from build123d import *

# Parameters (mm, degrees)
SKETCH2_R          = 3.5
CUT_EXTRUDE1_DEPTH = 69.058798109
SKETCH3_R          = 7
CUT_EXTRUDE2_DEPTH = 10
SKETCH3_3_R        = 2.5
CUT_EXTRUDE3_DEPTH = 72.637978754
FILLET1_R          = 1


with BuildPart() as part:
    # Sketch1 → Revolve1 (revolve)
    with BuildSketch(Plane(origin=(0, 0, 0), x_dir=(0, 0, -1), z_dir=(1, 0, 0))):
        Polygon((0, 33), (-14, 33), (-14, 46), (6, 46), (6, 12), (16, 12), (16, 0), (0, 0), align=None)
    revolve(axis=Axis((0, 0, -16), (0, 0, 1)))

    # Sketch2 → Cut-Extrude1 (cut, through all)
    with BuildSketch(Plane(origin=(0, 0, -6), x_dir=(-1, 0, 0), z_dir=(0, 0, -1))):
        with Locations(Location((19.5, -33.774990748, 0), (0, 0, 90))):
            Circle(SKETCH2_R)
        with Locations(Location((-19.5, -33.774990748, 0), (0, 0, 90))):
            Circle(SKETCH2_R)
        with Locations(Location((-39, 0, 0), (0, 0, 90))):
            Circle(SKETCH2_R)
        with Locations(Location((-19.5, 33.774990748, 0), (0, 0, 90))):
            Circle(SKETCH2_R)
        with Locations(Location((19.5, 33.774990748, 0), (0, 0, 90))):
            Circle(SKETCH2_R)
        with Locations(Location((39, 0, 0), (0, 0, 90))):
            Circle(SKETCH2_R)
    extrude(amount=-CUT_EXTRUDE1_DEPTH, mode=Mode.SUBTRACT)

    # Sketch3 → Cut-Extrude2 (cut)
    with BuildSketch(Plane(origin=(0, 0, -16), x_dir=(-1, 0, 0), z_dir=(0, 0, -1))):
        with Locations(Location((0, 0, 0), (0, 0, 90))):
            Circle(SKETCH3_R)
    extrude(amount=-CUT_EXTRUDE2_DEPTH, mode=Mode.SUBTRACT)

    # Sketch3_3 → Cut-Extrude3 (cut, through all)
    with BuildSketch(Plane(origin=(0, 0, -16), x_dir=(-1, 0, 0), z_dir=(0, 0, -1))):
        with Locations(Location((0, 0, 0), (0, 0, 90))):
            Circle(SKETCH3_3_R)
    extrude(amount=-CUT_EXTRUDE3_DEPTH, mode=Mode.SUBTRACT)

    # Fillet1
    fillet1_edges = [part.edges().sort_by_distance(p)[0] for p in [
        (0, -46, -6),
    ]]
    fillet(fillet1_edges, radius=FILLET1_R)


solid = part.part
Input: part model. Units: mm. Frame: model coordinates. A direction names the side the tool comes from. Give positions to 0.01 mm unless a question says otherwise; leave off trailing zeros. Order: outer loops, then holes, each group sorted by start corner. A loop starts at its lowest first (then second) coordinate and runs counter-clockwise, first axis right, second up. Notation, with made-up numbers: (23.25, 10) - (70.25, 10) arc R18 ccw to (70.25, 23) - close; hole circle Ø3 at (8, -27.5). An arc over 180 degrees is marked (long way). Answer as a JSON object with one key per item and string values. Group by question number.
Q1. Cut plane C-C, the plane y = 0. Count the separate pieces of the cut face and the enclosed holes in it, then the cut area to 3 significant figures.
Q2. Cut plane A-A, the plane x = 0. Output: boundary loops of the cut face in (y, z), then the cut area to 3 significant figures.
Q3. Mould query, pull axis Y, two halves, no side actions, for faces 4 (the face through (-0.53, -11.99, -11.07)), 5 (the face through (9, 9, -6)), 6 (the face through (-16.55, -31.89, 3.86)). Classes: pulls with the +Y half, pulls with the -Y half, needs draft (parallel to the pull), parting line crosses it, or undercut.
Q4. First-contact query: pin 1 Ø15.5 at (x, y) = (0.5, -1) entering from -Z; pin 2 Ø8 at (x, y) = (-19.5, -33.77) entering from -Z; pin 3 Ø12 at (x, z) = (-10, -11) entering from +Y; pin 4 Ø3 at (x, y) = (-9.5, 27.5) entering from +Z. Flat tips, straight axial feed; report the tip coordinate or a pass-through.
Q5. Cut plane B-B, the plane z = 6.5. Output: boundary loops of the cut face in (x, y) (3 decimals), then the cut area to 3 significant figures.
Q6. Line query: probe 1 along X at (y, z) = (0, 9.5); probe 2 along Z at (x, y) = (-9, -29.5); probe 3 along Y at (x, z) = (0, 9.5). Output: solid intervals per line, ascending.
Q7. Cut plane D-D, the plane z = -9.25. Output: boundary loops of the cut face in (x, y).
Q8. Set-up query: faces 1 (the face through (-6.834, -1.517, -11.07)), 2 (the face through (12.6, 30.5, 7.1)), 3 (the face through (21.87, 31.2, 3.86)). Return all of +Z, -Z, +X, -X, +Y, -Y with unobstructed straight access to the full face (end or side cutting, diameter ignored); none if empty.
Results:
{
 "1": {"separate pieces": "4", "enclosed holes": "0", "area": "706 mm^2"},
 "2": {"outline": "(-46, -5) arc R1 ccw to (-45, -6) - (-12, -6) - (-12, -16) - (-7, -16) - (-7, -6) - (-2.5, -6) - (-2.5, 0) - (-33, 0) - (-33, 14) - (-46, 14) - close; (2.5, -6) - (7, -6) - (7, -16) - (12, -16) - (12, -6) - (45, -6) arc R1 ccw to (46, -5) - (46, 14) - (33, 14) - (33, 0) - (2.5, 0) - close", "area": "986 mm^2"},
 "3": {"face 4": "parting line crosses it", "face 5": "needs draft", "face 6": "undercut"},
 "4": {"pin 1": "z = -16", "pin 2": "z = -6", "pin 3": "y = 45.24", "pin 4": "z = 0"},
 "5": {"outline": "circle Ø92 at (0, 0); hole circle Ø7 at (-39, 0); hole circle Ø66 at (0, 0); hole circle Ø7 at (-19.5, -33.775); hole circle Ø7 at (-19.5, 33.775); hole circle Ø7 at (19.5, -33.775); hole circle Ø7 at (19.5, 33.775); hole circle Ø7 at (39, 0)", "area": "3,000 mm^2"},
 "6": {"probe 1": "-46 to -42.5, -35.5 to -33, 33 to 35.5, 42.5 to 46", "probe 2": "-6 to 0", "probe 3": "-46 to -33, 33 to 46"},
 "7": {"outline": "circle Ø24 at (0, 0); hole circle Ø14 at (0, 0)"},
 "8": {"face 1": "-Z", "face 2": "+Z", "face 3": "+Z, -Z"}
}
